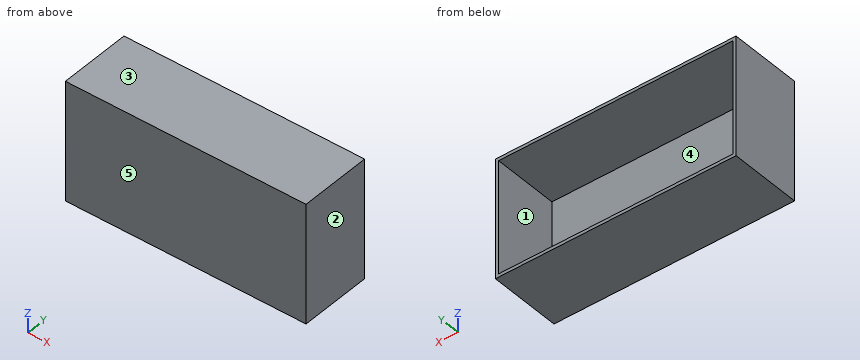
```python
from build123d import *

# Parameters (mm, degrees)
F0_W     = 806.45
F0_H     = 400.05
F1_DEPTH = 241.3
F2_W     = 784.86
F2_H     = 378.46
F3_DEPTH = 219.71


with BuildPart() as f1:
    # F0 (on Front) → F1 (new body)
    with BuildSketch(Plane.XZ):
        Rectangle(F0_W, F0_H)
    extrude(amount=F1_DEPTH)

    # F2 (on face) → F3 (cut)
    with BuildSketch(Plane(origin=(0, 0, 0), x_dir=(-1, 0, 0), z_dir=(0, 1, 0))):
        Rectangle(F2_W, F2_H)
    extrude(amount=-F3_DEPTH, mode=Mode.SUBTRACT)


solid = f1.part
```
Check sheet for the modelled part. Datum: model origin and axes. Units: mm. Face numbers are marked on the shaded views. A direction names the side the tool comes from. Round coordinates to 2 decimals unless told otherwise and drop trailing zeros. Loops run counter-clockwise (first coordinate to the right, second up) from the corner with the lowest first, then second, coordinate; pieces in that order, holes last. Notation, with made-up numbers: (59, 48) -> (98, 48) arc R23 ccw to (98, 73) -> close; hole circle Ø3 at (78, -14). An arc over 180 degrees is marked (long way). Answer in a Markdown table with one row per item.
Q1. Set-up check for the marked faces 4 and 5: record each of +Z, -Z, +X, -X, +Y, -Y from which the full face is reachable in a straight line by a thin tool's end or side.
Data:
| item | result |
|---|---|
| face 4 | +Y |
| face 5 | +Z, -Z, +X, -X, -Y |
Q2. Thickness scan on L1, parallel to Z at x = -89, y = -217.5 (3 decimals); L2, parallel to X at y = -133.5, z = 20.5 (3 decimals); L3, parallel to Y at x = -103.5, z = -55.5. Record the ranges inside material, lowest first.
Data:
| item | result |
|---|---|
| L1 | z = -200.025 to -189.23, 189.23 to 200.025 |
| L2 | x = -403.225 to -392.43, 392.43 to 403.225 |
| L3 | y = -241.3 to -219.71 |
Q3. Sectioned sample at B-B on z = 144. Enter the section's corners in (x, y) (3 decimals), then the cut area to 3 significant figures.
Data:
| item | result |
|---|---|
| outline | (-403.225, -241.3) -> (403.225, -241.3) -> (403.225, 0) -> (392.43, 0) -> (392.43, -219.71) -> (-392.43, -219.71) -> (-392.43, 0) -> (-403.225, 0) -> close |
| area | 22,200 mm^2 |
Q4. Sectioned sample at A-A on y = -58. Enter the section's corners in (x, z) (3 decimals), then the cut area to 3 significant figures.
Data:
| item | result |
|---|---|
| outline | (-403.225, -200.025) -> (403.225, -200.025) -> (403.225, 200.025) -> (-403.225, 200.025) -> close; hole (-392.43, -189.23) -> (392.43, -189.23) -> (392.43, 189.23) -> (-392.43, 189.23) -> close |
| area | 25,600 mm^2 |
Q5. Release check for a two-part mould opening along Z. For the marked faces 1, 2 and 3 record: released by +Z, released by -Z, zero draft, split by the parting line, or undercut.
Data:
| item | result |
|---|---|
| face 1 | undercut |
| face 2 | zero draft |
| face 3 | released by +Z |
Q6. Go/stop test with a flat-tipped pin: P1, Ø4, axis at x = 117, z = 63, coming from the +Y side. Record where the tip stops, or that it passes through.
Data:
| item | result |
|---|---|
| P1 | stops at y = -219.71 |
Q7. Sectioned sample at C-C on x = -118.5. Enter the section's corners in (y, z) (3 decimals), then the cut area to 3 significant figures.
Data:
| item | result |
|---|---|
| outline | (-241.3, -200.025) -> (0, -200.025) -> (0, -189.23) -> (-219.71, -189.23) -> (-219.71, 189.23) -> (0, 189.23) -> (0, 200.025) -> (-241.3, 200.025) -> close |
| area | 13,400 mm^2 |
